```python
from build123d import *

# Parameters (mm, degrees)
SKETCH_1_R               = 170
EXTRUDE_1_DEPTH          = 8
SKETCH_5_R               = 4
CUT_EXTRUDE_4_DEPTH      = 10
PATTERN_CIRCULAR_3_COUNT = 4
SKETCH_7_R               = 160
SKETCH_7_R_2             = 157
CUT_EXTRUDE_5_DEPTH      = 2
FILLET_1_R               = 0.3
SKETCH_9_R               = 7
CUT_EXTRUDE_7_DEPTH      = 10
PATTERN_CIRCULAR_5_COUNT = 2


with BuildPart() as part:
    # 草图1 → 凸台-拉伸1 (new body)
    with BuildSketch(Plane(origin=(0, 0, 0), x_dir=(0, 0, -1), z_dir=(1, 0, 0))):
        Circle(SKETCH_1_R)
    extrude(amount=EXTRUDE_1_DEPTH)

    # 草图5 → 切除-拉伸4 (cut)
    with BuildSketch(Plane(origin=(8, 0, 0), x_dir=(0, 0, -1), z_dir=(1, 0, 0))):
        with Locations((-91.923881554, 91.923881554)):
            Circle(SKETCH_5_R)
    cut_extrude_4 = extrude(amount=-CUT_EXTRUDE_4_DEPTH, mode=Mode.SUBTRACT)

    # 阵列(圆周)3: 切除-拉伸4 ×4 about axis
    pattern_circular_3_axis = Axis((0, 0, 0), (1, 0, 0))
    for i in range(1, PATTERN_CIRCULAR_3_COUNT):
        add(cut_extrude_4.rotate(pattern_circular_3_axis, i * 360 / PATTERN_CIRCULAR_3_COUNT), mode=Mode.SUBTRACT)

    # 草图7 → 切除-拉伸5 (cut)
    with BuildSketch(Plane(origin=(8, 0, 0), x_dir=(0, 0, -1), z_dir=(1, 0, 0))):
        Circle(SKETCH_7_R)
        Circle(SKETCH_7_R_2, mode=Mode.SUBTRACT)
    extrude(amount=-CUT_EXTRUDE_5_DEPTH, mode=Mode.SUBTRACT)

    # 圆角1
    fillet_1_edges = [part.edges().sort_by_distance(p)[0] for p in [
        (0, 0, 170),
        (8, 0, 170),
    ]]
    fillet(fillet_1_edges, radius=FILLET_1_R)

    # 草图9 → 切除-拉伸7 (cut)
    with BuildSketch(Plane(origin=(8, 0, 0), x_dir=(0, 0, -1), z_dir=(1, 0, 0))):
        with Locations((42.426406871, -42.426406871)):
            Circle(SKETCH_9_R)
    cut_extrude_7 = extrude(amount=-CUT_EXTRUDE_7_DEPTH, mode=Mode.SUBTRACT)

    # 阵列(圆周)5: 切除-拉伸7 ×2 about axis
    pattern_circular_5_axis = Axis((0, 0, 0), (1, 0, 0))
    for i in range(1, PATTERN_CIRCULAR_5_COUNT):
        add(cut_extrude_7.rotate(pattern_circular_5_axis, i * 360 / PATTERN_CIRCULAR_5_COUNT), mode=Mode.SUBTRACT)


solid = part.part
```
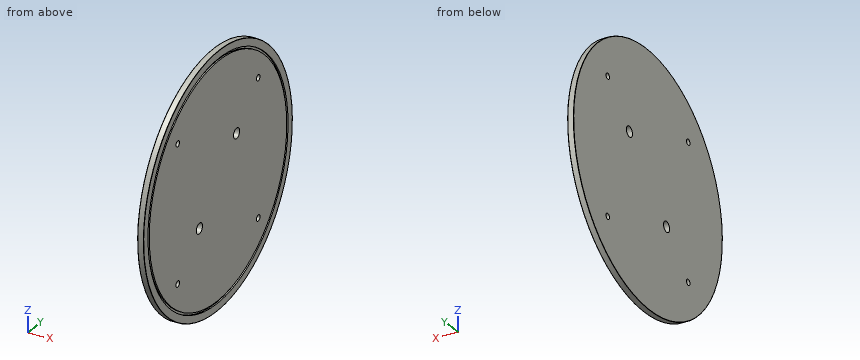
Here's how the part is built. I have some questions about the finished solid (model axes, mm). Round coordinates to 2 decimals unless told otherwise and drop trailing zeros. Loops run counter-clockwise (first coordinate to the right, second up) from the corner with the lowest first, then second, coordinate; pieces in that order, holes last.
1. Will this pin go through, and if not, where does the flat tip stop? pin 1 (2 mm diameter, centred on y = 78.5, z = 65, fed in from -X).
Answers:
pin 1: stops at x = 0
2. Suppose I cut it at A-A, the plane x = 2.25. Please give me the cut outline in (y, z), and give its area (3 significant figures).
Answers:
outline: circle Ø340 at (0, 0); hole circle Ø8 at (-91.92, -91.92); hole circle Ø8 at (-91.92, 91.92); hole circle Ø14 at (-42.43, -42.43); hole circle Ø14 at (42.43, 42.43); hole circle Ø8 at (91.92, -91.92); hole circle Ø8 at (91.92, 91.92)
area: 90,300 mm2
3. If I drill on probe 1 along Y at (x, z) = (6.9, 0); probe 2 along Y at (x, z) = (7, -30); probe 3 along Z at (x, y) = (7.25, 23), over which ranges is the centre line in solid material (lowest first)?
Answers:
probe 1: y = -170 to -160, -157 to 157, 160 to 170
probe 2: y = -167.33 to -157.16, -154.11 to 154.11, 157.16 to 167.33
probe 3: z = -168.44 to -158.34, -155.31 to 155.31, 158.34 to 168.44
